from build123d import *

# Parameters (mm, degrees)
SKETCH009_W             = 84
SKETCH009_H             = 70
PAD002_DEPTH            = 2
SKETCH010_W             = 2
SKETCH010_H             = 7
PAD003_DEPTH            = 2
SKETCH012_W             = 8
SKETCH012_H             = 6.8
PAD004_DEPTH            = 4
SKETCH013_W             = 7
SKETCH013_H             = 6
PAD005_DEPTH            = 4
SKETCH011_W             = 8
SKETCH011_H             = 6.8
PAD006_DEPTH            = 4
SKETCH014_R             = 1.15
POCKET002_DEPTH         = 81.001
SKETCH016_R             = 1.15
POCKET003_DEPTH         = 8.501
SKETCH018_W             = 11.5
SKETCH018_H             = 11.5
POCKET004_DEPTH         = 5
POCKET005_DEPTH         = 5
POCKET006_DEPTH         = 5
SKETCH021_W             = 1
SKETCH021_H             = 7
PAD007_DEPTH            = 1
SKETCH022_W             = 9
SKETCH022_H             = 10
POCKET007_DEPTH         = 0.4
FILLET_R                = 3
BODY002_PITCH_ANGLE     = -90
BODY002_PLACEMENT_ANGLE = 90
PAD001_DEPTH            = 35
SKETCH007_W             = 11.5
SKETCH007_H             = 11.5
POCKET001_DEPTH         = 13
FILLET001_R             = 3
SKETCH025_W             = 6.5
SKETCH025_H             = 9
SKETCH025_W_2           = 9
SKETCH025_H_2           = 6.5
POCKET008_DEPTH         = 8


with BuildPart() as back:
    # Sketch009 → Pad002 (new body)
    with BuildSketch(Plane.XY):
        Rectangle(SKETCH009_W, SKETCH009_H)
    extrude(amount=PAD002_DEPTH)

    # Sketch010 (on Face6 of Pad002) → Pad003 (join)
    with BuildSketch(Plane.XY.offset(2)):
        with Locations((-38, -1)):
            Rectangle(SKETCH010_W, SKETCH010_H)
        Polygon((-21, 32), (39, 32), (39, -4), (37, -4), (37, 30), (-21, 30), align=None)
    extrude(amount=PAD003_DEPTH)

    # Sketch012 (on Face15 of Pad003) → Pad004 (join)
    with BuildSketch(Plane.YZ.offset(39)):
        with Locations((0, 5.4)):
            Rectangle(SKETCH012_W, SKETCH012_H)
    extrude(amount=-PAD004_DEPTH)

    # Sketch013 (on Face9 of Pad004) → Pad005 (join)
    with BuildSketch(Plane(origin=(-39, 0, 0), x_dir=(0, -1, 0), z_dir=(-1, 0, 0))):
        with Locations((1, 5)):
            Rectangle(SKETCH013_W, SKETCH013_H)
    extrude(amount=-PAD005_DEPTH)

    # Sketch011 (on Face16 of Pad003) → Pad006 (join)
    with BuildSketch(Plane(origin=(0, 32, 0), x_dir=(-1, 0, 0), z_dir=(0, 1, 0))):
        with Locations((-29, 5.4)):
            Rectangle(SKETCH011_W, SKETCH011_H)
        with Locations((14, 5.4)):
            Rectangle(SKETCH011_W, SKETCH011_H)
    extrude(amount=-PAD006_DEPTH)

    # Sketch014 (on Face44 of Pad006) → Pocket002 (cut, through all)
    with BuildSketch(Plane.YZ.offset(39)):
        with Locations((0, 5)):
            Circle(SKETCH014_R)
    extrude(amount=-POCKET002_DEPTH, mode=Mode.SUBTRACT)

    # Sketch016 → Pocket003 (cut, through all)
    with BuildSketch(Plane.XZ.offset(-26.5)):
        with Locations((-13, 5)):
            Circle(SKETCH016_R)
        with Locations((30, 5)):
            Circle(SKETCH016_R)
    extrude(amount=-POCKET003_DEPTH, mode=Mode.SUBTRACT)

    # Sketch018 (on Face5 of Pocket003) → Pocket004 (cut)
    with BuildSketch(Plane.XY.offset(2)):
        with Locations((0, 17.75)):
            Rectangle(SKETCH018_W, SKETCH018_H)
    extrude(amount=-POCKET004_DEPTH, mode=Mode.SUBTRACT)

    # Sketch019 (on Face31 of Pocket004) → Pocket005 (cut)
    with BuildSketch(Plane.XZ.offset(-28)):
        Polygon((29.125944, 9.042901), (33.258869, 4.499726), (33.258869, 9.042901), align=None)
    extrude(amount=-POCKET005_DEPTH, mode=Mode.SUBTRACT)

    # Sketch020 (on Face36 of Pocket005) → Pocket006 (cut)
    with BuildSketch(Plane(origin=(35, 0, 0), x_dir=(0, -1, 0), z_dir=(-1, 0, 0))):
        Polygon((2.77547, 8.938441), (6.386171, 3.079567), (6.386171, 8.938441), align=None)
    extrude(amount=-POCKET006_DEPTH, mode=Mode.SUBTRACT)

    # Sketch021 (on Face40 of Pocket006) → Pad007 (join)
    with BuildSketch(Plane.XY.offset(8)):
        with Locations((-38.5, -1)):
            Rectangle(SKETCH021_W, SKETCH021_H)
    extrude(amount=PAD007_DEPTH)

    # Sketch022 (on Face5 of Pocket005) → Pocket007 (cut)
    with BuildSketch(Plane.XY.offset(2)):
        with Locations((-30.3, 30)):
            Rectangle(SKETCH022_W, SKETCH022_H)
    extrude(amount=-POCKET007_DEPTH, mode=Mode.SUBTRACT)

    # Fillet
    fillet_edges = [back.edges().sort_by_distance(p)[0] for p in [
        (42, 35, 1),
        (-42, 35, 1),
    ]]
    fillet(fillet_edges, radius=FILLET_R)


with BuildPart() as back_1:
    # Body002 pitch: moved
    add(back.part.rotate(Axis((0, 0, 0), (0, 1, 0)), BODY002_PITCH_ANGLE))


with BuildPart() as back_2:
    # Body002 placement: moved
    add(back_1.part.rotate(Axis((0, 0, 0), (0, 0, 1)), BODY002_PLACEMENT_ANGLE))


with BuildPart() as curve:
    # Sketch006 → Pad001 (new body, symmetric)
    with BuildSketch(Plane(origin=(0, 0, 0), x_dir=(0, 0, -1), z_dir=(1, 0, 0))):
        with BuildLine():
            ThreePointArc((-42, 3.9), (0, 0.945451), (42, 3.9))
            Line((42, -0.1), (42, 3.9))
            Line((-42, -0.1), (42, -0.1))
            Line((-42, 3.9), (-42, -0.1))
        make_face()
    extrude(amount=PAD001_DEPTH, both=True)

    # Sketch007 (on Face3 of Pad001) → Pocket001 (cut)
    with BuildSketch(Plane.XZ.offset(0.1)):
        with Locations((-17.75, 0)):
            Rectangle(SKETCH007_W, SKETCH007_H)
    extrude(amount=-POCKET001_DEPTH, mode=Mode.SUBTRACT)

    # Fillet001
    fillet001_edges = [curve.edges().sort_by_distance(p)[0] for p in [
        (-35, 1.9, -42),
        (-35, 1.9, 42),
    ]]
    fillet(fillet001_edges, radius=FILLET001_R)

    # Boolean: union Back
    add(back_2.part)

    # Sketch025 (on Face32 of Boolean) → Pocket008 (cut, symmetric)
    with BuildSketch(Plane.XZ.offset(2)):
        with Locations((-28.75, 0)):
            Rectangle(SKETCH025_W, SKETCH025_H)
        with Locations((-15.55, 13.625)):
            Rectangle(SKETCH025_W_2, SKETCH025_H_2)
        with Locations((-2.05, 0)):
            Rectangle(SKETCH025_W, SKETCH025_H)
        with Locations((-15.55, -13.625)):
            Rectangle(SKETCH025_W_2, SKETCH025_H_2)
    extrude(amount=POCKET008_DEPTH, both=True, mode=Mode.SUBTRACT)


solid = curve.part
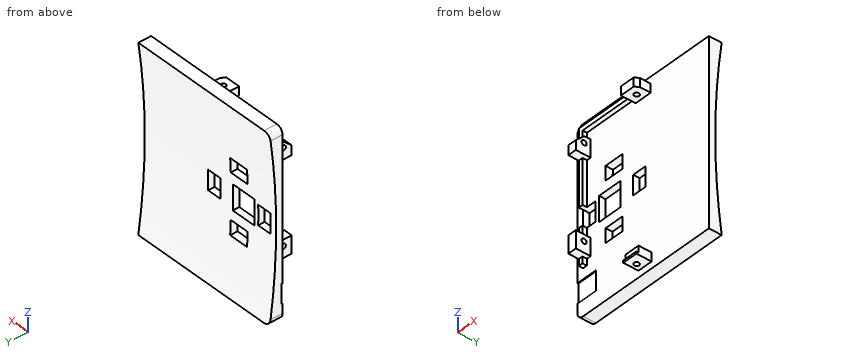
Can you work these out from the model? Positions are in its coordinate system, mm. Give positions to 0.01 mm unless a question says otherwise; leave off trailing zeros. Order: outer loops, then holes, each group sorted by start corner. A loop starts at its lowest first (then second) coordinate and runs counter-clockwise, first axis right, second up. Notation, with made-up numbers: M 70,15 L 83,15 A20 cw 83,53 Z; hole C -9,82.25 d8. An arc over 180 degrees is marked long. Use one line per item in the form item = value. Start each with the question number.
Item 1: If we section it at A-A (x = 0): Write out the boundary of the cut face in (y, z), then the cut area to 3 significant figures.
Item 2: If we section it at D-D (z = 12.5): Write out the boundary of the cut face in (x, y), then the cut area to 3 significant figures.
Item 3: If we section it at C-C (z = -2): Write out the boundary of the cut face in (x, y), then the cut area to 3 significant figures.
Item 4: Will these pins go through, and if not, where does the flat tip stop? pin 1 Ø2 at (x, z) = (-30, 26.5) entering from -Y; pin 2 Ø3 at (y, z) = (-4.5, 36.5) entering from -X; pin 3 Ø4 at (x, z) = (-5.5, 8.5) entering from -Y.
Item 5: If we section it at B-B (x = -29): Write out the boundary of the cut face in (y, z).
Item 6: If I drill on line 1 along X through (y, z) = (0.75, 13); line 2 along Z through (x, y) = (-29, -1.5); line 3 along Y through (x, z) = (17, -34), over which ranges is the centre line in solid material (lowest first)?
Outcome:
q1.outline = M -9,-39 L -6.15,-39 L -6.15,-35 L -8,-35 L -8,-38 L -9,-38 Z; M -8.8,35 L -6.15,35 L -6.15,39 L -8.8,39 Z; M -3.85,-39 L -2,-39 L -2,-42 L 3.9,-42 A300 cw 0.98,-4.5 L -2,-4.5 L -2,-35 L -3.85,-35 Z; M -3.85,35 L -2,35 L -2,4.5 L 0.98,4.5 A300 cw 3.9,42 L -2,42 L -2,39 L -3.85,39 Z
q1.area = 337 mm2
q2.outline = M -35,-2 L -32,-2 L -32,-4 L -30,-4 L -30,-2 L -20.05,-2 L -20.05,1.21 L -35,1.21 Z; M -11.05,-2 L 35,-2 L 35,1.21 L -11.05,1.21 Z
q2.area = 200 mm2
q3.outline = M -35,-2 L -32,-2 L -32,0.95 L -35,0.95 Z; M -25.5,-2 L -23.5,-2 L -23.5,0.95 L -25.5,0.95 Z; M -12,-2 L -5.3,-2 L -5.3,0.95 L -12,0.95 Z; M 1.2,-2 L 35,-2 L 35,0.95 L 1.2,0.95 Z
q3.area = 134 mm2
q4.pin_1 = -8.8
q4.pin_2 = -32
q4.pin_3 = -2
q5.outline = M -8.8,-18 L -2,-18 L -2,-25.8 L -1.6,-25.8 L -1.6,-34.8 L -2,-34.8 L -2,-42 L 3.9,-42 A300 cw 0.98,-4.5 L -2,-4.5 L -2,-10 L -8.8,-10 Z; M -8.8,25 L -2,25 L -2,4.5 L 0.98,4.5 A300 cw 3.9,42 L -2,42 L -2,39 L -4,39 L -4,37 L -2,37 L -2,33 L -4.78,33 L -8.8,29.35 Z; hole C -5,-13 d2.3; hole C -5,30 d2.3
q6.line_1 = -35 to -20.05, -11.05 to 35
q6.line_2 = -42 to -4.5, 4.5 to 42
q6.line_3 = -2 to 2.88
